CAD build for the part. Positions are in the model's coordinates, mm. A direction names the side the tool comes from. Round coordinates to 2 decimals unless told otherwise and drop trailing zeros. Write each loop counter-clockwise with the first axis right and the second up, starting at its lowest first coordinate (ties: lowest second). Pieces come first, ordered by that corner, then holes. Notation, with made-up numbers: (39.25, -29.75) -> (93.25, -29.75) arc R29 ccw to (93.25, 0.25) -> close; hole circle Ø11 at (22, 23). An arc over 180 degrees is marked (long way). Put each result on its own line as item: value. Start each with the question number.
1. Flat gauge pins, fed straight in: P1, Ø1.1, axis at y = 4, z = 12, coming from the +X side; P2, Ø0.8, axis at y = 4, z = -12, coming from the -X side; P3, Ø0.8, axis at x = 6.5, y = 3.5, coming from the +Z side; P4, Ø2.5, axis at x = 7, z = 12.5, coming from the -Y side. Where does each tip first touch, or does it go through?
2. Saw through at C-C on x = -3.5. List the corners of the cut face in (y, z).
3. Saw through at D-D on y = 4. List the corners of the cut face in (x, z), and give its area (3 significant figures).
4. Saw through at A-A on y = 2.15. List the corners of the cut face in (x, z), and give its area (3 significant figures).
5. Drill centre lines: line 1 (X direction, y = 1, z = -12.5); line 2 (X direction, y = 3.35, z = -1); line 3 (Y direction, x = -7.5, z = 10). Where is each one in solid material? Low to high. Write a range as from..to.
6. Saw through at B-B on z = 6. List the corners of the cut face in (x, y).
7. Pull direction X, two halves, no side cores. Call faces 6 (the cylindrical face through (9.4, 1.52, 14.93)), 7 (the cylindrical face through (-9.43, 1.52, 14.9)), 8 (the flat face through (2, 4, -12.5)), 9 (the cylindrical face through (-8.464, 1.521, -12.825)): pulls with the +X half, pulls with the -X half, needs draft (parallel to the pull), parting line crosses it, or undercut.
8. 3-axis set-ups, long thin cutter, end or side, ignore diameter. For faces 1 (the flat face through (0, 1, -15.5)), 2 (the flat face through (7, 4, -1)), 3 (the flat face through (-7, 4, 1)), 4 (the cylindrical face through (4.57, 3.99, 10.1)), 5 (the cylindrical face through (-4.57, 3.99, -10.1)): which of +Z, -Z, +X, -X, +Y, -Y reach the whole face in a straight line?
from build123d import *

# Parameters (mm, degrees)
CROQUIS1_W              = 20
CROQUIS1_H              = 31
SALIENTE_EXTRUIR1_DEPTH = 3
REDONDEO1_R             = 2
SALIENTE_EXTRUIR2_DEPTH = 2
CROQUIS3_R              = 1.5
CORTAR_EXTRUIR1_DEPTH   = 4


with BuildPart() as part:
    # Croquis1 → Saliente-Extruir1 (new body)
    with BuildSketch(Plane(origin=(0, 0, 0), x_dir=(1, 0, 0), z_dir=(0, 1, 0))):
        Rectangle(CROQUIS1_W, CROQUIS1_H)
    extrude(amount=SALIENTE_EXTRUIR1_DEPTH)

    # Redondeo1
    redondeo1_edges = [part.edges().sort_by_distance(p)[0] for p in [
        (10, 1.5, 15.5),
        (-10, 1.5, 15.5),
        (-10, 1.5, -15.5),
        (10, 1.5, -15.5),
    ]]
    fillet(redondeo1_edges, radius=REDONDEO1_R)

    # Croquis2 → Saliente-Extruir2 (add)
    with BuildSketch(Plane(origin=(0, 3, 0), x_dir=(1, 0, 0), z_dir=(0, 1, 0))):
        with BuildLine():
            Line((-7, -12.5), (4, -12.5))
            Line((4, -12.5), (4, -11.5))
            ThreePointArc((4, -11.5), (4.585786438, -10.085786438), (6, -9.5))
            Line((6, -9.5), (7, -9.5))
            Line((7, -9.5), (7, 12.5))
            Line((7, 12.5), (-4, 12.5))
            Line((-4, 12.5), (-4, 11.5))
            ThreePointArc((-4, 11.5), (-4.585786438, 10.085786438), (-6, 9.5))
            Line((-6, 9.5), (-7, 9.5))
            Line((-7, 9.5), (-7, -12.5))
        make_face()
    extrude(amount=SALIENTE_EXTRUIR2_DEPTH)

    # Croquis3 → Cortar-Extruir1 (cut)
    with BuildSketch(Plane(origin=(0, 3, 0), x_dir=(1, 0, 0), z_dir=(0, 1, 0))):
        with Locations(Location((-7, 12.5, 0), (0, 0, 270))):
            Circle(CROQUIS3_R)
        with Locations(Location((7, -12.5, 0), (0, 0, 270))):
            Circle(CROQUIS3_R)
    extrude(amount=-CORTAR_EXTRUIR1_DEPTH, mode=Mode.SUBTRACT)


solid = part.part
Return value:
1. P1: stops at x = 4
1. P2: stops at x = -4
1. P3: stops at z = 9.5
1. P4: passes through
2. outline: (0, -15.5) -> (3, -15.5) -> (3, -12.5) -> (5, -12.5) -> (5, 12.5) -> (3, 12.5) -> (3, 15.5) -> (0, 15.5) -> close
3. outline: (-7, -9.5) -> (-6, -9.5) arc R2 cw to (-4, -11.5) -> (-4, -12.5) -> (7, -12.5) -> (7, 9.5) -> (6, 9.5) arc R2 cw to (4, 11.5) -> (4, 12.5) -> (-7, 12.5) -> close
3. area: 334 mm^2
4. outline: (-10, -13.5) arc R2 ccw to (-8, -15.5) -> (8, -15.5) arc R2 ccw to (10, -13.5) -> (10, 13.5) arc R2 ccw to (8, 15.5) -> (-8, 15.5) arc R2 ccw to (-10, 13.5) -> close; hole circle Ø3 at (-7, -12.5); hole circle Ø3 at (7, 12.5)
4. area: 602 mm^2
5. line 1: x = -10..-8.5, -5.5..10
5. line 2: x = -7..7
5. line 3: y = 0..3
6. outline: (-10, 0) -> (10, 0) -> (10, 3) -> (7, 3) -> (7, 5) -> (-7, 5) -> (-7, 3) -> (-10, 3) -> close
7. face 6: pulls with the +X half
7. face 7: pulls with the -X half
7. face 8: needs draft
7. face 9: undercut
8. face 1: -Z, +X, -X, +Y, -Y
8. face 2: +Z, -Z, +X, +Y
8. face 3: +Z, -Z, -X, +Y
8. face 4: +Z, +X, +Y
8. face 5: -Z, -X, +Y
